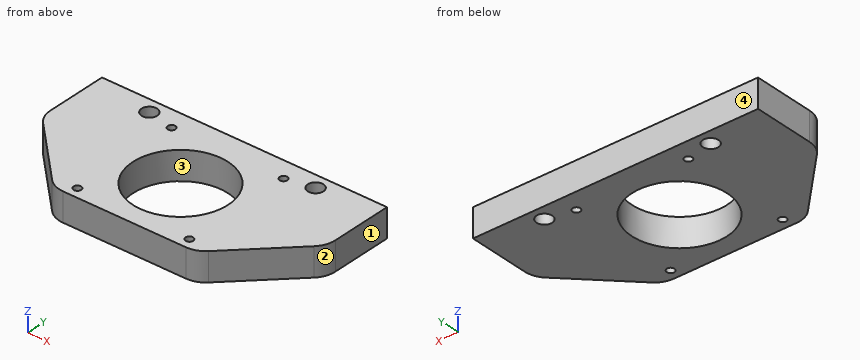
Autodesk Inventor part; units mm, degrees
ref_plane "YZ Plane" through (0, 0, 0) normal (1, 0, 0) x (0, 1, 0)
ref_plane "XZ Plane" through (0, 0, 0) normal (0, 1, 0) x (-1, 0, 0)
ref_plane "XY Plane" through (0, 0, 0) normal (0, 0, 1) x (1, 0, 0)
sketch "Sketch1" plane through (0, 0, 0) normal (0, 0, 1) x (1, 0, 0)
  line L0 (-60, -30) -> (60, -30)
  line L1 (60, -30) -> (60, 30)
  line L2 (60, 30) -> (-60, 30)
  line L3 (-60, 30) -> (-60, -30)
  line L4 (-60, -30) -> (60, 30) construction
  line L5 (60, -30) -> (-60, 30) construction
  point P0 (0, 0)
  dimension "d0" = 120
  dimension "d1" = 60
extrude "Extrusion1" add sketch "Sketch1" along normal blind 12
sketch "Sketch2" plane through (0, 0, 12) normal (0, 0, 1) x (1, 0, 0)
  line L0 (60, 30) -> (-60, 30)
  point P0 (0, 0)
  point P1 (0, -2)
  point P2 (0, 30)
  dimension "d4" = 32
hole "Hole1" at (0, -2, 12) direction (0, 0, -1) diameter 40 end through all
chamfer "Chamfer1" distance 30 angle 45 2 edges at (60, -30, 6) (-60, -30, 6)
sketch "Sketch3" plane through (0, 0, 12) normal (0, 0, 1) x (1, 0, 0)
  line L0 (60, 30) -> (-60, 30)
  point P0 (0, 0)
  point P1 (-35, 24)
  point P2 (35, 24)
  dimension "d15" = 6
  dimension "d16" = 70
  dimension "d17" = 35
hole "Hole2" at (-35, 24, 12) at (35, 24, 12) direction (0, 0, -1) diameter 6.6 end through all
sketch "Sketch4" plane through (0, 0, 12) normal (0, 0, 1) x (1, 0, 0)
  line L0 (-23.57, -25.57) -> (23.57, -25.57)
  line L1 (23.57, -25.57) -> (23.57, 21.57)
  line L2 (23.57, 21.57) -> (-23.57, 21.57)
  line L3 (-23.57, 21.57) -> (-23.57, -25.57)
  line L4 (-23.57, -25.57) -> (23.57, 21.57) construction
  line L5 (23.57, -25.57) -> (-23.57, 21.57) construction
  circle A0 centre (0, -2) radius 20
  dimension "d25" = 47.14
  dimension "d26" = 47.14
hole "Hole3" at (-23.57, 21.57, 12) at (23.57, 21.57, 12) at (23.57, -25.57, 12) at (-23.57, -25.57, 12) direction (0, 0, -1) diameter 3.242 end through all
fillet "Fillet1" radius 10 4 edges at (-30, -30, 6) (-60, 0, 6) (30, -30, 6) (60, 0, 6)
properties part number "Motorhalterung" material "Aluminum 6061"
Verification items for the finished model (mm, model axes). Face numbers are marked on the shaded views. Coordinates: 2 decimals unless noted, no trailing zeros. Order: outer loops, then holes, each group sorted by start corner. A loop starts at its lowest first (then second) coordinate and runs counter-clockwise, first axis right, second up. Notation, with made-up numbers: (79, 85.25) - (111, 85.25) arc R3 cw to (111, 90.25) - close; hole circle Ø5 at (55, 17.5). An arc over 180 degrees is marked (long way). Return JSON: item names as keys, results as strings.
(1) Section check A-A, the plane x = 0. Record the cut outline in (y, z), and give its area (3 significant figures).
Filled sheet:
{"outline": "(-30, 0) - (-22, 0) - (-22, 12) - (-30, 12) - close; (18, 0) - (30, 0) - (30, 12) - (18, 12) - close", "area": "240 mm^2"}
(2) Section check D-D, the plane z = 1.5. Record the cut outline in (x, y), and give its area (3 significant figures).
Filled sheet:
{"outline": "(-60, 4.14) arc R10 ccw to (-57.07, -2.93) - (-32.93, -27.07) arc R10 ccw to (-25.86, -30) - (25.86, -30) arc R10 ccw to (32.93, -27.07) - (57.07, -2.93) arc R10 ccw to (60, 4.14) - (60, 30) - (-60, 30) - close; hole circle Ø6.6 at (-35, 24); hole circle Ø3.24 at (-23.57, -25.57); hole circle Ø3.24 at (-23.57, 21.57); hole circle Ø40 at (0, -2); hole circle Ø3.24 at (23.57, -25.57); hole circle Ø3.24 at (23.57, 21.57); hole circle Ø6.6 at (35, 24)", "area": "4,930 mm^2"}
(3) Thickness scan on line 1 along Y through (x, z) = (-23.57, 3.5); line 2 along Y through (x, z) = (0, 6); line 3 along X through (y, z) = (-25.57, 2.75). Record the ranges inside material, lowest first.
Filled sheet:
{"line 1": "y = -30 to -27.19, -23.95 to 19.95, 23.19 to 30", "line 2": "y = -30 to -22, 18 to 30", "line 3": "x = -34.43 to -25.19, -21.95 to 21.95, 25.19 to 34.43"}
(4) Mould release check, pull along Y, two halves, no side actions. Record for the marked faces 1, 2, 3 and 4: pulls with the +Y half, pulls with the -Y half, needs draft (parallel to the pull), parting line crosses it, or undercut.
Filled sheet:
{"face 1": "needs draft", "face 2": "pulls with the -Y half", "face 3": "undercut", "face 4": "pulls with the +Y half"}
(5) Section check B-B, the plane y = -25.57. Record the cut outline in (x, z), and give its area (3 significant figures).
Filled sheet:
{"outline": "(-34.43, 0) - (-25.19, 0) - (-25.19, 12) - (-34.43, 12) - close; (-21.95, 0) - (21.95, 0) - (21.95, 12) - (-21.95, 12) - close; (25.19, 0) - (34.43, 0) - (34.43, 12) - (25.19, 12) - close", "area": "749 mm^2"}
(6) Section check C-C, the plane x = 23.57. Record the cut outline in (y, z), and give its area (3 significant figures).
Filled sheet:
{"outline": "(-30, 0) - (-27.19, 0) - (-27.19, 12) - (-30, 12) - close; (-23.95, 0) - (19.95, 0) - (19.95, 12) - (-23.95, 12) - close; (23.19, 0) - (30, 0) - (30, 12) - (23.19, 12) - close", "area": "642 mm^2"}
(7) Go/stop test with a flat-tipped pin: pin 1 (4 mm diameter, centred on x = 34, z = 10.5, fed in from -Y). Record where the tip stops, or that it passes through.
Filled sheet:
{"pin 1": "stops at y = -27.89"}
